```python
from build123d import *

# Parameters (mm, degrees)
BOSS_EXTRUDE1_DEPTH = 50.8
SKETCH2_W           = 25.4
SKETCH2_H           = 25.4
CUT_EXTRUDE1_DEPTH  = 90.090296329
FILLET1_R           = 1.27
SKETCH4_W           = 13.97
SKETCH4_H           = 22.86
CUT_EXTRUDE2_DEPTH  = 90.090296329
FILLET2_R           = 2.54


with BuildPart() as part:
    # Sketch1 → Boss-Extrude1 (new body)
    with BuildSketch(Plane.XY):
        with BuildLine():
            Line((33.252294453, 57.15), (45.72, 57.15))
            Line((45.72, 57.15), (45.72, 0))
            Line((45.72, 0), (0, 0))
            Line((0, 0), (0, 57.15))
            Line((0, 57.15), (12.467705547, 57.15))
            ThreePointArc((12.467705547, 57.15), (22.86, 43.434), (33.252294453, 57.15))
        make_face()
    extrude(amount=BOSS_EXTRUDE1_DEPTH)

    # Sketch2 → Cut-Extrude1 (cut, through all)
    with BuildSketch(Plane(origin=(45.72, 0, 0), x_dir=(0, 0, -1), z_dir=(1, 0, 0))):
        with Locations((-25.4, 12.7)):
            Rectangle(SKETCH2_W, SKETCH2_H)
    extrude(amount=-CUT_EXTRUDE1_DEPTH, mode=Mode.SUBTRACT)

    # Fillet1
    fillet1_edges = [part.edges().sort_by_distance(p)[0] for p in [
        (22.86, 25.4, 38.1),
        (22.86, 25.4, 12.7),
    ]]
    fillet(fillet1_edges, radius=FILLET1_R)

    # Sketch4 → Cut-Extrude2 (cut, through all)
    with BuildSketch(Plane.ZY):
        with Locations((43.815, 45.72)):
            Rectangle(SKETCH4_W, SKETCH4_H)
        with Locations((6.985, 45.72)):
            Rectangle(SKETCH4_W, SKETCH4_H)
    extrude(amount=-CUT_EXTRUDE2_DEPTH, mode=Mode.SUBTRACT)

    # Fillet2
    fillet2_edges = [part.edges().sort_by_distance(p)[0] for p in [
        (22.86, 34.29, 36.83),
        (22.86, 34.29, 50.8),
        (22.86, 34.29, 0),
        (22.86, 34.29, 13.97),
    ]]
    fillet(fillet2_edges, radius=FILLET2_R)


solid = part.part
```
Part model, mm, in its own coordinate system. A direction names the side the tool comes from. Coordinates: 2 decimals unless noted, no trailing zeros. Order: outer loops, then holes, each group sorted by start corner. A loop starts at its lowest first (then second) coordinate and runs counter-clockwise, first axis right, second up. Notation, with made-up numbers: (87, 49) - (102, 49) arc R28 cw to (102, 79) - close; hole circle Ø4 at (89, -5). An arc over 180 degrees is marked (long way). Return JSON: item names as keys, results as strings. Group by question number.
Item 1: Drill centre lines: probe 1 along Z at (x, y) = (25.5, 16.5); probe 2 along Z at (x, y) = (2.5, 37); probe 3 along Y at (x, z) = (22.86, 20.5). Where is each one in solid material? Low to high. Write a range as from..to.
Item 2: Which spindle directions (+Z, -Z, +X, -X, +Y, -Y) get a long thin tool onto all of the face, cutting with end or side? Do faces 4 (the face through (23, 12, 38.1)), 5 (the face through (23, 34.29, 44)), 6 (the face through (23, 42, 13.97)), 7 (the face through (23, 16, 50.8)). Say none if no direction does.
Item 3: Cut at D-D (y = 4). List the corners of the cut face in (x, z), plus the area to 3 significant figures.
Item 4: Pin check, flat tips, straight feed: pin 1 (22.5 mm diameter, centred on x = 19, y = 52, fed in from +Z); pin 2 (4 mm diameter, centred on x = 9.5, z = 10.5, fed in from +Y); pin 3 (2 mm diameter, centred on x = 22, y = 38, fed in from -Z). Stop position of each tip, or through.
Item 5: Cut at A-A (y = 50.5). List the corners of the cut face in (x, z), plus the area to 3 significant figures.
Item 6: Cut at B-B (x = 22.86). List the corners of the cut face in (y, z).
Item 7: Cut at C-C (z = 32.5). List the corners of the cut face in (x, y) (3 decimals).
Item 8: Pull direction X, two halves, no side cores. Call faces 1 (the face through (22.581, 43.438, 25.24)), 2 (the face through (0, 28, 25)), 3 (the face through (23, 34.29, 7)): pulls with the +X half, pulls with the -X half, needs draft (parallel to the pull), parting line crosses it, or undercut.
Check values:
{
 "1": {"probe 1": "z = 0..12.7, 38.1..50.8", "probe 2": "z = 13.97..36.83", "probe 3": "y = 25.4..43.43"},
 "2": {"face 4": "+X, -X, -Y", "face 5": "+Z, +X, -X, +Y", "face 6": "-Z, +X, -X, +Y", "face 7": "+Z, +X, -X, +Y, -Y"},
 "3": {"outline": "(0, 0) - (45.72, 0) - (45.72, 12.7) - (0, 12.7) - close; (0, 38.1) - (45.72, 38.1) - (45.72, 50.8) - (0, 50.8) - close", "area": "1,160 mm2"},
 "4": {"pin 1": "stops at z = 36.83", "pin 2": "stops at y = 34.53", "pin 3": "stops at z = 13.97"},
 "5": {"outline": "(0, 13.97) - (12.73, 13.97) - (12.73, 36.83) - (0, 36.83) - close; (32.99, 13.97) - (45.72, 13.97) - (45.72, 36.83) - (32.99, 36.83) - close", "area": "582 mm2"},
 "6": {"outline": "(0, 0) - (31.75, 0) arc R2.54 ccw to (34.29, 2.54) - (34.29, 11.43) arc R2.54 cw to (36.83, 13.97) - (43.43, 13.97) - (43.43, 36.83) - (36.83, 36.83) arc R2.54 cw to (34.29, 39.37) - (34.29, 48.26) arc R2.54 ccw to (31.75, 50.8) - (0, 50.8) - (0, 38.1) - (24.13, 38.1) arc R1.27 cw to (25.4, 36.83) - (25.4, 13.97) arc R1.27 cw to (24.13, 12.7) - (0, 12.7) - close"},
 "7": {"outline": "(0, 25.4) - (45.72, 25.4) - (45.72, 57.15) - (33.252, 57.15) arc R10.795 cw (long way) to (12.468, 57.15) - (0, 57.15) - close"},
 "8": {"face 1": "undercut", "face 2": "pulls with the -X half", "face 3": "needs draft"}
}
